Geometry: final body of the model. Coordinates: model frame, mm. Face numbers are marked on the shaded views. Round coordinates to 2 decimals unless told otherwise and drop trailing zeros. Order: outer loops, then holes, each group sorted by start corner. A loop starts at its lowest first (then second) coordinate and runs counter-clockwise, first axis right, second up. Notation, with made-up numbers: M -33.5,-4 L 3.5,-4 A13 ccw 3.5,1 Z; hole C 18.25,-3 d6. An arc over 180 degrees is marked long. Return JSON: item names as keys, results as strings. Group by question number.
Q1. Ray query, probe 1 along Y at (x, z) = (86.5, 40.5); probe 2 along X at (y, z) = (-10, 89); probe 3 along X at (y, z) = (-93, 45.5). Return the intervals inside material, ascending.
Q2. Cut plane B-B on x = 134.5. Output: boundary loops of the cut face in (y, z).
Q3. Contact query for flat-ended pins moving along their axis: pin 1 (8 mm diameter, centred on x = 100, y = -87.5, fed in from -Z); pin 2 (4 mm diameter, centred on y = -111, z = 23, fed in from +X); pin 3 (3 mm diameter, centred on x = 100, y = -36, fed in from +Z). Output: stop coordinate, or through.
Q4. Cut plane C-C on y = -55.5. Output: boundary loops of the cut face in (x, z), and give its area (3 significant figures).
Q5. Mould query, pull axis X, two halves, no side actions, for the marked faces 1, 2, 3 and 4. Classes: released by +X, released by -X, zero draft, split by the parting line, or undercut.
Q6. Cut plane A-A on y = -179. Output: boundary loops of the cut face in (x, z), and give its area (3 significant figures).
```python
from build123d import *

# Parameters (mm, degrees)
F1_DEPTH = 254
F2_T     = -2.5
F4_D     = 100


with BuildPart() as f1:
    # F0 (on Front) → F1 (new body)
    with BuildSketch(Plane.XZ):
        Polygon((-10.566324, 6.683148), (111.352801, 39.486691), (185.046107, 112.936161), (54.999065, 104.22466), align=None)
    extrude(amount=F1_DEPTH)

    # F2
    f2_openings = [f1.faces().sort_by_distance(p)[0] for p in [
        (120.022586, -127, 108.58041),
    ]]
    offset(amount=F2_T, openings=f2_openings)

    # F4 (through all)
    with Locations(Plane(origin=(-10.372185, 0, 6.971968), x_dir=(0, -1, 0), z_dir=(-0.829933, 0, 0.557864))):
        with Locations((142.56683, 67.633435)):
            Hole(F4_D / 2)


solid = f1.part
```
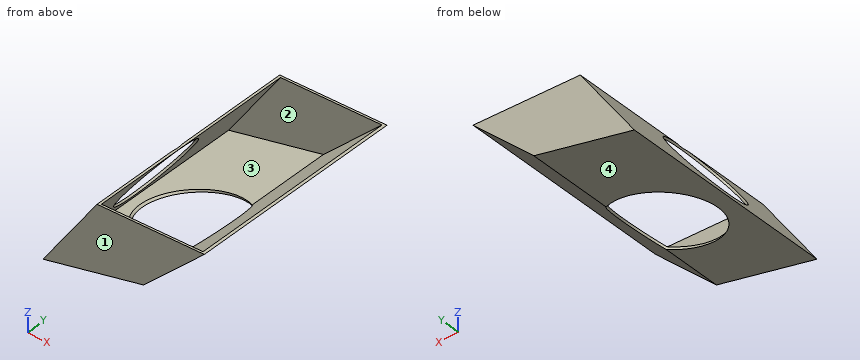
Result sheet:
{
 "1": {"probe 1": "y = -254 to -251.5, -2.5 to 0", "probe 2": "x = 44.77 to 47.78, 157.49 to 161.03", "probe 3": "x = 15.53 to 18.54, 113.84 to 117.39"},
 "2": {"outline": "M -254,62.56 L 0,62.56 L 0,109.55 L -2.5,109.55 L -2.5,66.09 L -251.5,66.09 L -251.5,109.55 L -254,109.55 Z"},
 "3": {"pin 1": "stops at z = 35.36", "pin 2": "stops at x = 4.76", "pin 3": "stops at z = 39.42"},
 "4": {"outline": "M -10.57,6.68 L 111.35,39.49 L 185.05,112.94 L 181.25,112.68 L 110.06,41.73 L -4.76,10.83 L 58.15,104.44 L 55,104.22 Z", "area": "850 mm²"},
 "5": {"face 1": "zero draft", "face 2": "undercut", "face 3": "undercut", "face 4": "released by +X"},
 "6": {"outline": "M -10.57,6.68 L 32.62,18.3 L 29.87,20.15 L -4.76,10.83 L 10.33,33.29 L 8.25,34.68 Z; M 46.46,91.52 L 48.54,90.13 L 58.15,104.44 L 55,104.22 Z; M 114.28,45.94 L 116.4,44.51 L 185.05,112.94 L 181.25,112.68 Z", "area": "457 mm²"}
}
